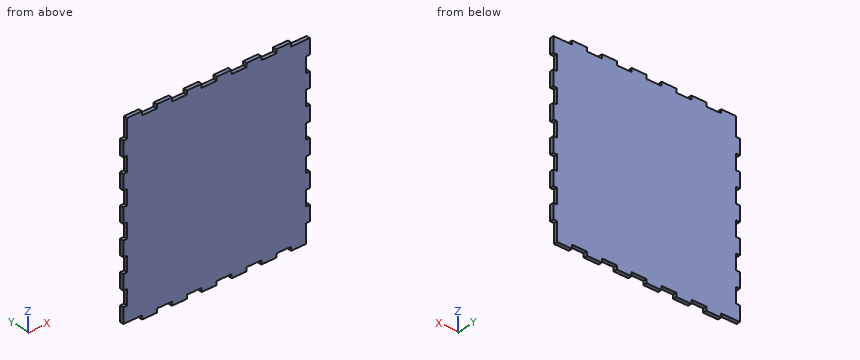
from build123d import *

# Parameters (mm, degrees)
BOSS_EXTRUDE1_DEPTH = 6.35


with BuildPart() as part:
    # Sketch1 → Boss-Extrude1 (new body)
    with BuildSketch(Plane(origin=(0, 0, 0), x_dir=(1, 0, 0), z_dir=(0, 1, 0))):
        Polygon((-65.292450766, -101.6), (-39.892450766, -101.6), (-39.892450766, -107.95), (-14.492450766, -107.95), (-14.492450766, -101.6), (10.907549234, -101.6), (10.907549234, -107.95), (36.307549234, -107.95), (36.307549234, -101.6), (61.707549234, -101.6), (61.707549234, -107.95), (87.107549234, -107.95), (87.107549234, -101.6), (112.507549234, -101.6), (112.507549234, -107.95), (137.907549234, -107.95), (137.907549234, -101.6), (163.307549234, -101.6), (163.307549234, -107.95), (188.707549234, -107.95), (188.707549234, -101.6), (220.457549234, -101.6), (220.457549234, -76.2), (214.107549234, -76.2), (214.107549234, -50.8), (220.457549234, -50.8), (220.457549234, -25.4), (214.107549234, -25.4), (214.107549234, 0), (220.457549234, 0), (220.457549234, 25.4), (214.107549234, 25.4), (214.107549234, 50.8), (220.457549234, 50.8), (220.457549234, 76.2), (214.107549234, 76.2), (214.107549234, 101.6), (220.457549234, 101.6), (220.457549234, 127), (214.107549234, 127), (214.107549234, 152.4), (220.457549234, 152.4), (220.457549234, 177.8), (214.107549234, 177.8), (214.107549234, 209.55), (188.707549234, 209.55), (188.707549234, 203.2), (163.307549234, 203.2), (163.307549234, 209.55), (137.907549234, 209.55), (137.907549234, 203.2), (112.507549234, 203.2), (112.507549234, 209.55), (87.107549234, 209.55), (87.107549234, 203.2), (61.707549234, 203.2), (61.707549234, 209.55), (36.307549234, 209.55), (36.307549234, 203.2), (10.907549234, 203.2), (10.907549234, 209.55), (-14.492450766, 209.55), (-14.492450766, 203.2), (-39.892450766, 203.2), (-39.892450766, 209.55), (-65.292450766, 209.55), (-65.292450766, 203.2), (-97.042450766, 203.2), (-97.042450766, 177.8), (-90.692450766, 177.8), (-90.692450766, 152.4), (-97.042450766, 152.4), (-97.042450766, 127), (-90.692450766, 127), (-90.692450766, 101.6), (-97.042450766, 101.6), (-97.042450766, 76.2), (-90.692450766, 76.2), (-90.692450766, 50.8), (-97.042450766, 50.8), (-97.042450766, 25.4), (-90.692450766, 25.4), (-90.692450766, 0), (-97.042450766, 0), (-97.042450766, -25.4), (-90.692450766, -25.4), (-90.692450766, -50.8), (-97.042450766, -50.8), (-97.042450766, -76.2), (-90.692450766, -76.2), (-90.692450766, -107.95), (-65.292450766, -107.95), align=None)
    extrude(amount=BOSS_EXTRUDE1_DEPTH)


solid = part.part
The listing builds one solid part. Answer for the finished solid, in the listing's coordinates (mm). Coordinates: 2 decimals unless noted, no trailing zeros. Write each loop counter-clockwise with the first axis right and the second up, starting at its lowest first coordinate (ties: lowest second). Pieces come first, ordered by that corner, then holes. Notation, with made-up numbers: (-38, 81.25) - (17, 81.25) arc R25 ccw to (17, 108.25) - close; hole circle Ø11 at (22.25, 39.5). An arc over 180 degrees is marked (long way). Answer as CSV lines item,"result".
1. Find section B-B (z = 85). Give the vertices of the cut face in (x, y).
Computed values:
outline,"(-90.69, 0) - (220.46, 0) - (220.46, 6.35) - (-90.69, 6.35) - close"
2. Given P1, Ø3, axis at x = -93.5, y = 4, coming from the -Z side; P2, Ø3, axis at y = 3, z = -207, coming from the +X side; P3, Ø1.5, axis at y = 2.5, z = -109, coming from the -X side, each flat-ended and moving along its own axis, determine where each tip first touches the part or whether it passes through.
Computed values:
P1,"stops at z = -203.2"
P2,"stops at x = 214.11"
P3,"stops at x = -90.69"
3. Straight lines are drawn through the part: line 1 (X direction, y = 2.5, z = -133); line 2 (Z direction, x = 22, y = 1.5); line 3 (Z direction, x = 53.5, y = 2.75). For each, find the intervals that lie inside material, in ascending order. Write a range as [from, to].
Computed values:
line 1,"x = [-97.04, 214.11]"
line 2,"z = [-203.2, 107.95]"
line 3,"z = [-209.55, 101.6]"
4. Find section A-A (x = 45). Give the vertices of the cut face in (y, z), plus the area to 3 significant figures.
Computed values:
outline,"(0, -209.55) - (6.35, -209.55) - (6.35, 101.6) - (0, 101.6) - close"
area,"1,980 mm²"
